Can you work these out from the model? Positions are in its coordinate system, mm. Round coordinates to 2 decimals unless told otherwise and drop trailing zeros. Order: outer loops, then holes, each group sorted by start corner. A loop starts at its lowest first (then second) coordinate and runs counter-clockwise, first axis right, second up. Notation, with made-up numbers: (46, -34) - (97, -34) arc R12 cw to (97, -30) - close; hole circle Ø2 at (58, 11). An arc over 180 degrees is marked (long way). Write item = value, one per line.
Autodesk Inventor part; units mm, degrees
ref_plane "YZ Plane" through (0, 0, 0) normal (1, 0, 0) x (0, 1, 0)
ref_plane "XZ Plane" through (0, 0, 0) normal (0, 1, 0) x (-1, 0, 0)
ref_plane "XY Plane" through (0, 0, 0) normal (0, 0, 1) x (1, 0, 0)
sketch "Эскиз1" plane through (0, 0, 0) normal (0, 0, 1) x (1, 0, 0)
  circle A0 centre (0, 0) radius 1.5
  dimension "d0" = 3
extrude "Выдавливание1" add sketch "Эскиз1" along normal blind 51.25
sketch "Эскиз2" plane through (0, 0, 51.25) normal (0, 0, 1) x (1, 0, 0)
  line L0 (-1.5, -1) -> (1.5, -1)
  line L1 (1.5, -1) -> (1.5, 1)
  line L2 (1.5, 1) -> (-1.5, 1)
  line L3 (-1.5, 1) -> (-1.5, -1)
  line L4 (-1.5, -1) -> (1.5, 1) construction
  line L5 (1.5, -1) -> (-1.5, 1) construction
  circle A0 centre (0, 0) radius 1.5
  point P0 (-1.118, 1)
  point P1 (1.118, 1)
  dimension "d3" = 2
extrude "Выдавливание2" cut sketch "Эскиз2" against normal blind 8 contours A0 L2
sketch "Эскиз3" plane through (0, 0, 0) normal (0, 0, -1) x (-1, 0, 0)
  arc A0 (1.118, 1) -> (-1.118, 1) centre (0, 0) ccw
  line L0 (-1.118, 1) -> (1.118, 1)
extrude "Выдавливание3" cut sketch "Эскиз3" against normal blind 5
equation "\"Радиус_гибки\" = Толщина"
equation "\"Ширина_просечки\" = Толщина"
equation "\"Глубина_просечки\" = 0.5 * Толщина"
equation "\"Размер_просечки\" = 4 * Толщина"
equation "\"Мин_остаток\" = 2 * Толщина"
equation "\"Радиус_перехода\" = Радиус_гибки"
equation "\"Радиус_Якоби\" = Толщина"
equation "\"Размер_зазора\" = Толщина"
properties part number "Ось 3мм задняя"
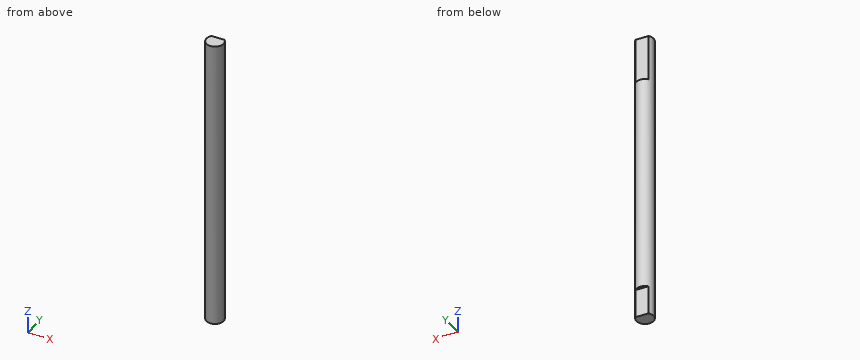
(1) If we section it at A-A (x = 0): Write out the boundary of the cut face in (y, z), plus the area to 3 significant figures.
Computed:
outline = (-1.5, 0) - (1, 0) - (1, 5) - (1.5, 5) - (1.5, 43.25) - (1, 43.25) - (1, 51.25) - (-1.5, 51.25) - close
area = 147 mm^2
(2) Will this pin go through, and if not, where does the flat tip stop? P1, Ø0.7, axis at x = 0, z = 1.5, coming from the +Y side.
Computed:
P1 = 1
(3) If we section it at B-B (z = 42): Write out the boundary of the cut face in (x, y).
Computed:
outline = circle Ø3 at (0, 0)
(4) If we section it at D-D (z = 48.5): Write out the boundary of the cut face in (x, y), plus the area to 3 significant figures.
Computed:
outline = (-1.12, 1) arc R1.5 ccw (long way) to (1.12, 1) - close
area = 6.29 mm^2
(5) If I drill on line 1 (Y direction, x = -1, z = 37); line 2 (X direction, y = 0.1, z = 10); line 3 (Z direction, x = -0.1, y = 1.3), over which ranges is the centre line in solid material (lowest first)? Write a range as from..to.
Computed:
line_1 = -1.12..1.12
line_2 = -1.5..1.5
line_3 = 5..43.25
(6) If we section it at C-C (y = -0.55): Write out the boundary of the cut face in (x, z), plus the area to 3 significant figures.
Computed:
outline = (-1.4, 0) - (1.4, 0) - (1.4, 51.25) - (-1.4, 51.25) - close
area = 143 mm^2
